Verification items for the finished model (mm, model axes). Face numbers are marked on the shaded views. Round coordinates to 2 decimals unless told otherwise and drop trailing zeros. Order: outer loops, then holes, each group sorted by start corner. A loop starts at its lowest first (then second) coordinate and runs counter-clockwise, first axis right, second up. Notation, with made-up numbers: (79, 75) -> (87, 75) arc R6 cw to (87, 85) -> close; hole circle Ø9 at (-10.75, 11). An arc over 180 degrees is marked (long way). Put each result on its own line as item: value.
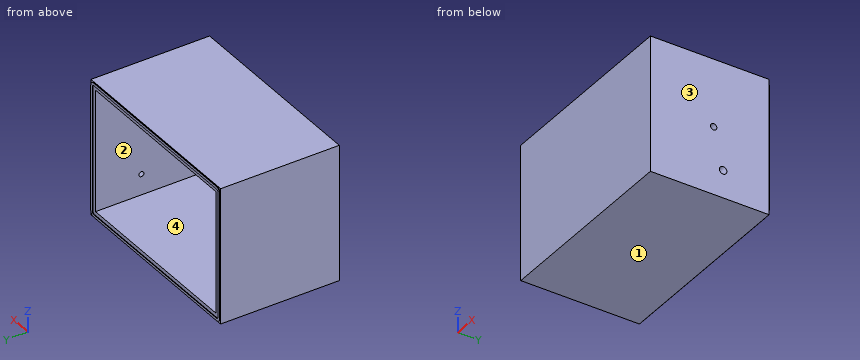
from build123d import *

# Parameters (mm, degrees)
SKETCH1_W           = 496.824
SKETCH1_H           = 342.9
BOSS_EXTRUDE1_DEPTH = 17.4625
BOSS_EXTRUDE2_START = -17.4625
SKETCH2_W           = 496.824
SKETCH2_H           = 342.9
SKETCH2_W_2         = 461.899
SKETCH2_H_2         = 307.975
BOSS_EXTRUDE2_DEPTH = 301
SKETCH11_W          = 461.899
SKETCH11_H          = 307.975
CUT_EXTRUDE2_DEPTH  = 1.5875
SKETCH30_R          = 9.525
CUT_EXTRUDE4_DEPTH  = 17.4625
CUT_EXTRUDE4_TAPER  = 10.304
SKETCH34_W          = 496.824
SKETCH34_H          = 342.9
CUT_EXTRUDE5_DEPTH  = 1.5875
CUT_EXTRUDE6_REACH  = 498.824
SKETCH35_R          = 8.001


with BuildPart() as part:
    # Sketch1 → Boss-Extrude1 (new body)
    with BuildSketch(Plane(origin=(0, 0, 0), x_dir=(1, 0, 0), z_dir=(0, 1, 0))):
        Rectangle(SKETCH1_W, SKETCH1_H)
    extrude(amount=BOSS_EXTRUDE1_DEPTH)

    # Sketch2 → Boss-Extrude2 (add)
    with BuildSketch(Plane(origin=(0, 17.4625, 0), x_dir=(1, 0, 0), z_dir=(0, 1, 0)).offset(BOSS_EXTRUDE2_START)):
        Rectangle(SKETCH2_W, SKETCH2_H)
        Rectangle(SKETCH2_W_2, SKETCH2_H_2, mode=Mode.SUBTRACT)
    extrude(amount=BOSS_EXTRUDE2_DEPTH)

    # Sketch11 → Cut-Extrude2 (cut)
    with BuildSketch(Plane(origin=(0, 301, 0), x_dir=(1, 0, 0), z_dir=(0, 1, 0))):
        with BuildLine():
            Line((235.3945, 163.5125), (-235.3945, 163.5125))
            ThreePointArc((-235.3945, 163.5125), (-238.986602448, 162.024602448), (-240.4745, 158.4325))
            Line((-240.4745, 158.4325), (-240.4745, -158.4325))
            ThreePointArc((-240.4745, -158.4325), (-238.986602448, -162.024602448), (-235.3945, -163.5125))
            Line((-235.3945, -163.5125), (235.3945, -163.5125))
            ThreePointArc((235.3945, -163.5125), (238.986602448, -162.024602448), (240.4745, -158.4325))
            Line((240.4745, -158.4325), (240.4745, 158.4325))
            ThreePointArc((240.4745, 158.4325), (238.986602448, 162.024602448), (235.3945, 163.5125))
        make_face()
        Rectangle(SKETCH11_W, SKETCH11_H, mode=Mode.SUBTRACT)
    extrude(amount=-CUT_EXTRUDE2_DEPTH, mode=Mode.SUBTRACT)

    # Sketch30 → Cut-Extrude4 (cut)
    with BuildSketch(Plane(origin=(248.412, 0, 0), x_dir=(0, 0, -1), z_dir=(1, 0, 0))):
        with Locations((101.6, 183.525)):
            Circle(SKETCH30_R)
    extrude(amount=-CUT_EXTRUDE4_DEPTH, taper=CUT_EXTRUDE4_TAPER, mode=Mode.SUBTRACT)

    # Sketch34 → Cut-Extrude5 (cut)
    with BuildSketch(Plane(origin=(0, 301, 0), x_dir=(1, 0, 0), z_dir=(0, 1, 0))):
        Rectangle(SKETCH34_W, SKETCH34_H)
        with BuildLine():
            Line((-235.3945, -169.8625), (235.3945, -169.8625))
            ThreePointArc((235.3945, -169.8625), (243.476730509, -166.514730509), (246.8245, -158.4325))
            Line((246.8245, -158.4325), (246.8245, 158.4325))
            ThreePointArc((246.8245, 158.4325), (243.476730509, 166.514730509), (235.3945, 169.8625))
            Line((235.3945, 169.8625), (-235.3945, 169.8625))
            ThreePointArc((-235.3945, 169.8625), (-243.476730509, 166.514730509), (-246.8245, 158.4325))
            Line((-246.8245, 158.4325), (-246.8245, -158.4325))
            ThreePointArc((-246.8245, -158.4325), (-243.476730509, -166.514730509), (-235.3945, -169.8625))
        make_face(mode=Mode.SUBTRACT)
    extrude(amount=-CUT_EXTRUDE5_DEPTH, mode=Mode.SUBTRACT)

    # Sketch35 → Cut-Extrude6 (cut, up to next)
    with BuildSketch(Plane(origin=(248.412, 0, 0), x_dir=(0, 0, -1), z_dir=(1, 0, 0)), mode=Mode.PRIVATE) as cut_extrude6_sk1:
        with Locations((0, 159.7125)):
            Circle(SKETCH35_R)
    cut_extrude6_tool1 = extrude(cut_extrude6_sk1.sketch, amount=-CUT_EXTRUDE6_REACH, mode=Mode.PRIVATE) & part.part
    add(cut_extrude6_tool1.solids().sort_by_distance((248.412, 159.7125, 0))[0], mode=Mode.SUBTRACT)


solid = part.part
Item 1: Section check D-D on z = 46.5. Record the boundary of the cut face in (x, y).
Check sheet entries:
outline: (-248.41, 0) -> (248.41, 0) -> (248.41, 299.41) -> (246.82, 299.41) -> (246.82, 301) -> (240.47, 301) -> (240.47, 299.41) -> (230.95, 299.41) -> (230.95, 17.46) -> (-230.95, 17.46) -> (-230.95, 299.41) -> (-240.47, 299.41) -> (-240.47, 301) -> (-246.82, 301) -> (-246.82, 299.41) -> (-248.41, 299.41) -> close
Item 2: Release check for a two-part mould opening along Z. For the marked faces 1, 2, 3 and 4 record: +Z half, -Z half, draft (parallel to the pull), parting line (faces both ways), or undercut.
Check sheet entries:
face 1: -Z half
face 2: undercut
face 3: draft
face 4: undercut
Item 3: Section check A-A on z = 0. Record the boundary of the cut face in (x, y).
Check sheet entries:
outline: (-248.41, 0) -> (248.41, 0) -> (248.41, 151.71) -> (230.95, 151.71) -> (230.95, 17.46) -> (-230.95, 17.46) -> (-230.95, 299.41) -> (-240.47, 299.41) -> (-240.47, 301) -> (-246.82, 301) -> (-246.82, 299.41) -> (-248.41, 299.41) -> close; (230.95, 167.71) -> (248.41, 167.71) -> (248.41, 299.41) -> (246.82, 299.41) -> (246.82, 301) -> (240.47, 301) -> (240.47, 299.41) -> (230.95, 299.41) -> close
Item 4: Section check B-B on x = -4. Record the boundary of the cut face in (y, z), then the cut area to 3 significant figures.
Check sheet entries:
outline: (0, -171.45) -> (299.41, -171.45) -> (299.41, -169.86) -> (301, -169.86) -> (301, -163.51) -> (299.41, -163.51) -> (299.41, -153.99) -> (17.46, -153.99) -> (17.46, 153.99) -> (299.41, 153.99) -> (299.41, 163.51) -> (301, 163.51) -> (301, 169.86) -> (299.41, 169.86) -> (299.41, 171.45) -> (0, 171.45) -> close
area: 15,900 mm^2
Item 5: Gauge pin test, flat ends, axial feed: pin 1 Ø0.8 at (y, z) = (300, 25.5) entering from +X; pin 2 Ø1.3 at (x, y) = (-77, 300) entering from +Z; pin 3 Ø6 at (x, z) = (-136.5, -52) entering from +Y; pin 4 Ø1.3 at (y, z) = (300.5, 44.5) entering from -X. Record the tip position at first contact, or that the pin passes through.
Check sheet entries:
pin 1: stops at x = 246.82
pin 2: stops at z = 171.45
pin 3: stops at y = 17.46
pin 4: stops at x = -246.82
Item 6: Section check C-C on y = 48. Record the boundary of the cut face in (x, z).
Check sheet entries:
outline: (-248.41, -171.45) -> (248.41, -171.45) -> (248.41, 171.45) -> (-248.41, 171.45) -> close; hole (-230.95, -153.99) -> (230.95, -153.99) -> (230.95, 153.99) -> (-230.95, 153.99) -> close
Item 7: Material ranges on L1, parallel to Z at x = -58, y = 270.5; L2, parallel to X at y = 65.5, z = -85; L3, parallel to Y at x = 241.25, z = 0, recorded low to high. Write a range as [from, to].
Check sheet entries:
L1: z = [-171.45, -153.99], [153.99, 171.45]
L2: x = [-248.41, -230.95], [230.95, 248.41]
L3: y = [0, 151.71], [167.71, 301]
